CAD build for the part. Positions are in the model's coordinates, mm. Coordinates: 2 decimals unless noted, no trailing zeros. Loops run counter-clockwise (first coordinate to the right, second up) from the corner with the lowest first, then second, coordinate; pieces in that order, holes last. Notation, with made-up numbers: (24, 40.25) -> (68, 40.25) arc R17 cw to (68, 44.25) -> close; hole circle Ø11 at (-38.75, 86.25). An arc over 180 degrees is marked (long way). Answer as CSV lines item,"result". Start each with the question number.
Autodesk Fusion 360 part; units mm, degrees
sketch "Side Panel" plane through (0, 0, 0) normal (1, 0, 0) x (0, 1, 0)
  line L0 (0, 0) -> (195, 0)
  line L1 (195, 0) -> (195, 520)
  line L2 (195, 520) -> (-0.3488, 600)
  line L3 (-0.3488, 600) -> (-0.3488, 510)
  line L4 (-0.3488, 510) -> (90, 473)
  line L5 (90, 473) -> (25, 345)
  line L6 (25, 345) -> (-65, 345)
  line L7 (-65, 345) -> (-65, 270)
  line L8 (-65, 270) -> (0, 270)
  line L9 (0, 270) -> (0, 0)
  dimension "d7" = 600
  dimension "d10" = 195
  dimension "d12" = 520
  dimension "d14" = 90
  dimension "d16" = 105
  dimension "d18" = 270
  dimension "d20" = 75
  dimension "d22" = 37
  dimension "d27" = 260
  dimension "d28" = 90
  dimension "d31" = 345
extrude "Extrude1" add sketch "Side Panel" along normal blind 6 makes body 1
fillet "Fillet1" radius 8 10 edges at (3, -65, 345) (3, 25, 345) (3, 90, 473) (3, -0.3488, 510) (3, -0.3488, 600) (3, 195, 520) (3, -65, 270) (3, 0, 270) (3, 0, 0) (3, 195, 0) on bodies 1
sketch "Paint border" plane through (6, 0, 0) normal (1, 0, 0) x (0, 1, 0)
  arc A0 (187, 0) -> (195, 8) centre (187, 8) ccw
  line L0 (195, 8) -> (195, 514.6313)
  arc A1 (195, 514.6313) -> (190.0318, 522.0346) centre (187, 514.6313) ccw
  line L1 (190.0318, 522.0346) -> (10.683, 595.4822)
  arc A2 (10.683, 595.4822) -> (-0.3488, 588.079) centre (7.6512, 588.079) ccw
  line L2 (-0.3488, 588.079) -> (-0.3488, 515.3687)
  arc A3 (-0.3488, 515.3687) -> (4.6194, 507.9654) centre (7.6512, 515.3687) ccw
  line L3 (4.6194, 507.9654) -> (81.9699, 476.2885)
  arc A4 (86.0711, 465.263) -> (81.9699, 476.2885) centre (78.9381, 468.8853) ccw
  line L4 (86.0711, 465.263) -> (27.2231, 349.3778)
  arc A5 (20.0901, 345) -> (27.2231, 349.3778) centre (20.0901, 353) ccw
  line L5 (20.0901, 345) -> (-57, 345)
  arc A6 (-57, 345) -> (-65, 337) centre (-57, 337) ccw
  line L6 (-65, 337) -> (-65, 278)
  arc A7 (-65, 278) -> (-57, 270) centre (-57, 278) ccw
  line L7 (-57, 270) -> (-8, 270)
  arc A8 (0, 262) -> (-8, 270) centre (-8, 262) ccw
  line L8 (0, 262) -> (0, 8)
  arc A9 (0, 8) -> (8, 0) centre (8, 8) ccw
  line L9 (8, 0) -> (187, 0)
  line L10 (10, 6) -> (185, 6)
  line L11 (10, 6) -> (10, 280)
  line L12 (10, 280) -> (-55, 280)
  line L13 (-55, 280) -> (-55, 335)
  line L14 (-55, 335) -> (31.1374, 335)
  line L15 (9.6512, 516.7108) -> (103.8274, 478.1434)
  line L16 (31.1374, 335) -> (103.8274, 478.1434)
  line L17 (187.0159, 512.4636) -> (185, 6)
  line L18 (9.6512, 585.0987) -> (187.0159, 512.4636)
  line L19 (9.6512, 585.0987) -> (9.6512, 516.7108)
  dimension "d32" = 6
  dimension "d33" = 10
  dimension "d34" = 10
  dimension "d35" = 10
  dimension "d36" = 10
  dimension "d37" = 10
  dimension "d41" = 10
  dimension "d42" = 10
  dimension "d43" = 10
  dimension "d44" = 10
extrude "Extrude2" cut sketch "Paint border" against normal blind 0.1 bodies 1
mirror "Mirror1" about plane through (0, 0, 0) normal (1, 0, 0) of bodies 1 makes body 2
hidden bodies 1
equation "MDFThickness = 6 mm"
equation "filletRadius = 8 mm"
equation "d3 = MDFThickness"
equation "d6 = filletRadius"
equation "d7 = totaHeight"
equation "totaHeight = 600 mm"
equation "baseWidth = 195 mm"
equation "d10 = baseWidth"
equation "backHight = 520 mm"
equation "d12 = backHight"
equation "namePanelHeight = 90 mm"
equation "d14 = namePanelHeight"
equation "neckWidth = 105 mm"
equation "d16 = neckWidth"
equation "bottomFrontHeight = 270 mm"
equation "d18 = bottomFrontHeight"
equation "controlPanelHeight = 75 mm"
equation "d20 = controlPanelHeight"
equation "namePanelFrontDipHeight = 37 mm"
equation "d22 = namePanelFrontDipHeight"
equation "controlPanelTopWidth = 90 mm"
equation "controlPanelTotalWidth = 260 mm"
equation "d27 = controlPanelTotalWidth"
equation "d28 = controlPanelTopWidth"
equation "d31 = bottomFrontHeight + controlPanelHeight"
Q1. Saw through at A-A (y = 61.5). List the corners of the cut face in (x, z).
Q2. Saw through at D-D (x = -3.1). List the corners of the cut face in (y, z).
Q3. Probe probe 1 along Z at (x, y) = (-5.45, -19); probe 2 along Z at (x, y) = (-2.55, 45.5); probe 3 along Y at (x, z) = (-4.8, 246.5). List the from-to ranges inside material, lowest first. Write a range as from..to.
Q4. Two-plate mould, pull along Z, no slides. Class faces 1 (the flat face through (-2.909, 56.235, 406.509)), 2 (the flat face through (0, 96, 302)), 3 (the flat face through (-2.909, 43.836, 491.905)), 4 (the flat face through (-2.909, 99.102, 559.273)): pulls with the +Z half, pulls with the -Z half, needs draft (parallel to the pull), parting line crosses it, or undercut.
Q5. Pin check, flat tip, straight feed: pin 1 Ø3 at (x, y) = (-2, -24) entering from -Z. Stop position of the tip, or through.
Q6. Saw through at C-C (z = 420). List the corners of the cut face in (x, y), and give its area (3 significant figures).
Q7. Saw through at B-B (y = 134). List the corners of the cut face in (x, z), and give its area (3 significant figures).
Ans:
1,outline,"(-6, 6) -> (-5.9, 6) -> (-5.9, 0) -> (0, 0) -> (0, 416.88) -> (-5.9, 416.88) -> (-5.9, 394.79) -> (-6, 394.79) -> close; (-6, 495.48) -> (-5.9, 495.48) -> (-5.9, 484.67) -> (0, 484.67) -> (0, 574.67) -> (-5.9, 574.67) -> (-5.9, 563.87) -> (-6, 563.87) -> close"
2,outline,"(-65, 278) arc R8 ccw to (-57, 270) -> (-8, 270) arc R8 cw to (0, 262) -> (0, 8) arc R8 ccw to (8, 0) -> (187, 0) arc R8 ccw to (195, 8) -> (195, 514.63) arc R8 ccw to (190.03, 522.03) -> (10.68, 595.48) arc R8 ccw to (-0.35, 588.08) -> (-0.35, 515.37) arc R8 ccw to (4.62, 507.97) -> (81.97, 476.29) arc R8 cw to (86.07, 465.26) -> (27.22, 349.38) arc R8 cw to (20.09, 345) -> (-57, 345) arc R8 ccw to (-65, 337) -> close"
3,probe 1,"z = 270..345"
3,probe 2,"z = 0..385.37, 491.22..581.22"
3,probe 3,"y = 0..195"
4,face 1,"undercut"
4,face 2,"needs draft"
4,face 3,"undercut"
4,face 4,"pulls with the +Z half"
5,pin 1,"stops at z = 270"
6,outline,"(-6, 74.3) -> (-5.9, 74.3) -> (-5.9, 63.09) -> (0, 63.09) -> (0, 195) -> (-5.9, 195) -> (-5.9, 186.65) -> (-6, 186.65) -> close"
6,area,"790 mm²"
7,outline,"(-6, 6) -> (-5.9, 6) -> (-5.9, 0) -> (0, 0) -> (0, 544.98) -> (-5.9, 544.98) -> (-5.9, 534.17) -> (-6, 534.17) -> close"
7,area,"3,270 mm²"
